For this review, take the finished solid that the model builds, in its own axes (mm). A direction names the side the tool comes from. Coordinates: 2 decimals unless noted, no trailing zeros. Loops run counter-clockwise (first coordinate to the right, second up) from the corner with the lowest first, then second, coordinate; pieces in that order, holes last. Notation, with made-up numbers: M 52.5,-26.75 L 68.5,-26.75 A31 cw 68.5,1.25 Z; hole C 56.25,31.25 d10. An arc over 180 degrees is marked long. Write item = value, one per line.
from build123d import *

# Parameters (mm, degrees)
F0_W       = 41.4983332157
F0_H       = 50.7746972144
F0_R       = 9.7686704189
F1_DEPTH   = 62.484
F2_R       = 15.6433873562
F1_FACE1_W = 41.4983332157
F1_FACE1_H = 50.7746972144
F1_FACE1_R = 9.7686704189
F3_DEPTH   = 108.966
F4_R       = 17.7535536274
F5_DEPTH   = 148.844
F6_R       = 6.8253458282
F7_DEPTH   = 248.92


with BuildPart() as f1:
    # F0 (on Front) → F1 (new body)
    with BuildSketch(Plane.XZ):
        with Locations((-87.555155158, -25.3873486072)):
            Rectangle(F0_W, F0_H)
        with Locations((-91.3773775101, -25.3873486072)):
            Circle(F0_R, mode=Mode.SUBTRACT)
    extrude(amount=-F1_DEPTH)

    # F2 (on face) + F1_face1 (on face) → F3 (join)
    with BuildSketch(Plane.XZ):
        with Locations((-91.3773775101, -25.3873486072)):
            Circle(F2_R)
    with BuildSketch(Plane(origin=(-86.9211204596, 62.484, -25.3873486072), x_dir=(1, 0, 0), z_dir=(0, 1, 0))):
        with Locations((-0.6340346985, 0)):
            Rectangle(F1_FACE1_W, F1_FACE1_H)
        with Locations((-4.4562570505, 0)):
            Circle(F1_FACE1_R, mode=Mode.SUBTRACT)
    extrude(amount=F3_DEPTH, dir=(0, -1, 0))

    # F4 (on face) → F5 (join)
    with BuildSketch(Plane(origin=(0, 62.484, 0), x_dir=(-1, 0, 0), z_dir=(0, 1, 0))):
        with Locations((91.3773775101, -25.3873486072)):
            Circle(F4_R)
    extrude(amount=F5_DEPTH)

    # F6 (on face) → F7 (join)
    with BuildSketch(Plane.XZ.offset(108.966)):
        with Locations((-91.3773775101, -25.3873486072)):
            Circle(F6_R)
    extrude(amount=-F7_DEPTH)


solid = f1.part
Q1. Machinability: for faces 1 (the face through (-76.927, -77.287, -31.379)), 2 (the face through (-89.3, 0, -18.7)), 3 (the face through (-74, 62.484, -19)), which of the approach directions +Z, -Z, +X, -X, +Y, -Y give a long, thin tool a straight path to every point of the face, cutting with its end or side? Answer none if there is none.
Solved:
face_1 = -Y
face_2 = none
face_3 = +Y
Q2. For pin 1 Ø1.5 at (y, z) = (176, -15.5) entering from -X; pin 2 Ø12 at (y, z) = (79.5, -18.5) entering from +X, all flat-tipped, find the tip position at first contact; note any pin that passes through.
Solved:
pin_1 = -106.6
pin_2 = -73.65
Q3. Draft analysis for pull direction Z (two halves, no side actions). For faces 4 (the face through (-88, 9, -50.775)), 5 (the face through (-98.196, 30.805, -25.087)), 6 (the face through (-88, 9, 0)), state which applies: +Z half, -Z half, draft (parallel to the pull), parting line (faces both ways), or undercut.
Solved:
face_4 = -Z half
face_5 = undercut
face_6 = +Z half
Q4. For line 1 along Z through (x, y) = (-93, 59); line 2 along Y through (x, z) = (-75, -13); line 3 along Y through (x, z) = (-95, -17), list the stretches that pass through material, from the lowest coordinate up.
Solved:
line_1 = -50.77 to -35.02, -32.02 to -18.76, -15.75 to 0
line_2 = -46.48 to 62.48
line_3 = -108.97 to 0, 62.48 to 211.33
Q5. Add section C-C (z = -46). Write out the cut boundary in (x, y), and give its area (3 significant figures).
Solved:
outline = M -108.3,-46.48 L -66.81,-46.48 L -66.81,62.48 L -108.3,62.48 Z
area = 4,520 mm²
Q6. Add section A-A (y = 9.5). Write out the cut boundary in (x, z).
Solved:
outline = M -108.3,-50.77 L -66.81,-50.77 L -66.81,0 L -108.3,0 Z; C -91.38,-25.39 d13.65; hole C -91.38,-25.39 d19.54
Q7. Add section B-B (x = -88.5). Write out the cut boundary in (y, z), and give its area (3 significant figures).
Solved:
outline = M -108.97,-40.76 L -46.48,-40.76 L -46.48,-50.77 L 62.48,-50.77 L 62.48,-42.91 L 211.33,-42.91 L 211.33,-7.87 L 62.48,-7.87 L 62.48,0 L -46.48,0 L -46.48,-10.01 L -108.97,-10.01 Z; hole M 0,-34.72 L 62.48,-34.72 L 62.48,-31.58 L 0,-31.58 Z; hole M 0,-19.2 L 62.48,-19.2 L 62.48,-16.05 L 0,-16.05 Z
area = 12,300 mm²
Q8. Add section D-D (y = -37). Write out the cut boundary in (x, z), and give its area (3 significant figures).
Solved:
outline = M -108.3,-50.77 L -66.81,-50.77 L -66.81,0 L -108.3,0 Z
area = 2,110 mm²
